from build123d import *

# Parameters (mm, degrees)
ESBO_O1_R                = 4
RESSALTO_EXTRUS_O1_DEPTH = 10
ESBO_O2_R                = 1.6
CORTE_EXTRUS_O1_DEPTH    = 10
RESSALTO_EXTRUS_O2_DEPTH = 2


with BuildPart() as part:
    # Esboço1 → Ressalto-extrusão1 (new body)
    with BuildSketch(Plane.XY):
        with BuildLine():
            Line((4, 53.65571123), (4, 6.34428877))
            ThreePointArc((4, 6.34428877), (0, -7.5), (-4, 6.34428877))
            Line((-4, 6.34428877), (-4, 53.65571123))
            ThreePointArc((-4, 53.65571123), (0, 67.5), (4, 53.65571123))
        make_face()
        with Locations((0, 60)):
            Circle(ESBO_O1_R, mode=Mode.SUBTRACT)
        Circle(ESBO_O1_R, mode=Mode.SUBTRACT)
    extrude(amount=RESSALTO_EXTRUS_O1_DEPTH)

    # Esboço2 → Corte-extrusão1 (cut)
    with BuildSketch(Plane.ZY.offset(4)):
        with Locations(Location((5, 30, 0), (0, 0, 270))):
            Circle(ESBO_O2_R)
    extrude(amount=-CORTE_EXTRUS_O1_DEPTH, mode=Mode.SUBTRACT)

    # Esboço3 → Ressalto-extrusão2 (add)
    with BuildSketch(Plane.XY.offset(10)):
        with BuildLine():
            Line((-4, 53.65571123), (-4, 6.34428877))
            ThreePointArc((-4, 6.34428877), (0, -7.5), (4, 6.34428877))
            Line((4, 6.34428877), (4, 53.65571123))
            ThreePointArc((4, 53.65571123), (0, 67.5), (-4, 53.65571123))
        make_face()
    extrude(amount=RESSALTO_EXTRUS_O2_DEPTH)


solid = part.part
Geometry check sheet. Reference: the model listing, model coordinates, mm. A direction names the side the tool comes from. Coordinates: 2 decimals unless noted, no trailing zeros. Order: outer loops, then holes, each group sorted by start corner. A loop starts at its lowest first (then second) coordinate and runs counter-clockwise, first axis right, second up. Notation, with made-up numbers: (33, -0.5) -> (58, -0.5) arc R20 ccw to (58, 13.5) -> close; hole circle Ø4 at (77, 35). An arc over 180 degrees is marked (long way). Use a Markdown table: item, result. Add a question column.
1. Go/stop test with flat-tipped pins: pin 1 Ø5 at (y, z) = (30, 5) entering from +X; pin 2 Ø1 at (x, z) = (-3.5, 5) entering from -Y; pin 3 Ø3 at (x, z) = (-5, 1.5) entering from -Y. Record where each tip stops, or that it passes through.
2. Cross-section at D-D (y = 0). Enter the section's corners in (x, z), and give its area (4 significant figures).
3. Set-up check for faces 1 (the face through (-4, 30, 7)), 2 (the face through (0, 60, 10)), 3 (the face through (0, 31, 12)): record each of +Z, -Z, +X, -X, +Y, -Y from which the full face is reachable in a straight line by a thin tool's end or side.
4. Cross-section at B-B (z = 5). Enter the section's corners in (x, y).
5. Material ranges on L1, parallel to Y at x = -0.25, z = 8.5; L2, parallel to Y at x = 2.75, z = 9.5; L3, parallel to Y at x = -2.75, z = 4.75, recorded low to high.
6. Cross-section at C-C (x = 0). Enter the section's corners in (y, z).
7. Cross-section at A-A (y = 30). Enter the section's corners in (x, z).
8. Mould release check, pull along Z, two halves, no side actions. Record for faces 4 (the face through (-0.06, 31.27, 4.03)), 5 (the face through (0, 31, 0)), 6 (the face through (-0.867, 56.095, 4.93)): pulls with the +Z half, pulls with the -Z half, needs draft (parallel to the pull), parting line crosses it, or undercut.
Filled sheet:
| question | item | result |
|---|---|---|
| 1 | pin 1 | x = 4 |
| 1 | pin 2 | y = -6.87 |
| 1 | pin 3 | y = -6.63 |
| 2 | outline | (-7.5, 0) -> (-4, 0) -> (-4, 10) -> (4, 10) -> (4, 0) -> (7.5, 0) -> (7.5, 12) -> (-7.5, 12) -> close |
| 2 | area | 100.0 mm2 |
| 3 | face 1 | +Z, -Z, -X |
| 3 | face 2 | -Z |
| 3 | face 3 | +Z, +X, -X, +Y, -Y |
| 4 | outline | (-4, 6.34) arc R7.5 ccw (long way) to (4, 6.34) -> (4, 28.4) -> (-4, 28.4) -> close; (-4, 31.6) -> (4, 31.6) -> (4, 53.66) arc R7.5 ccw (long way) to (-4, 53.66) -> close; hole circle Ø8 at (0, 0); hole circle Ø8 at (0, 60) |
| 5 | L1 | -7.5 to -3.99, 3.99 to 56.01, 63.99 to 67.5 |
| 5 | L2 | -6.98 to -2.9, 2.9 to 57.1, 62.9 to 66.98 |
| 5 | L3 | -6.98 to -2.9, 2.9 to 28.42, 31.58 to 57.1, 62.9 to 66.98 |
| 6 | outline | (-7.5, 0) -> (-4, 0) -> (-4, 10) -> (4, 10) -> (4, 0) -> (56, 0) -> (56, 10) -> (64, 10) -> (64, 0) -> (67.5, 0) -> (67.5, 12) -> (-7.5, 12) -> close; hole circle Ø3.2 at (30, 5) |
| 7 | outline | (-4, 0) -> (4, 0) -> (4, 3.4) -> (-4, 3.4) -> close; (-4, 6.6) -> (4, 6.6) -> (4, 12) -> (-4, 12) -> close |
| 8 | face 4 | undercut |
| 8 | face 5 | pulls with the -Z half |
| 8 | face 6 | needs draft |
